Build history of the part. All positions in model axes, mm. A direction names the side the tool comes from. Round coordinates to 2 decimals unless told otherwise and drop trailing zeros. Write each loop counter-clockwise with the first axis right and the second up, starting at its lowest first coordinate (ties: lowest second). Pieces come first, ordered by that corner, then holes. Notation, with made-up numbers: (3, 85.25) - (12, 85.25) arc R24 cw to (12, 104.25) - close; hole circle Ø2 at (85.25, 82). An arc over 180 degrees is marked (long way). Answer as a JSON object with one key per item and string values. Group by question number.
Item 1: Slice it at C-C, the plane x = -51. List the corners of the cut face in (y, z).
Item 2: Two-plate mould, pull along X, no slides. Class faces 1 (the flat face through (-111.898, -38, -30)), 2 (the cylindrical face through (-23.18, -48.6, -16.73)), 3 (the cylindrical face through (-61.11, -37.23, -30.02)), 4 (the flat face through (-10.298, -39, -25)): +X half, -X half, draft (parallel to the pull), parting line (faces both ways), or undercut.
Item 3: Slice it at B-B, the plane y = -33.5. List the corners of the cut face in (x, z).
Item 4: Slice it at D-D, the plane y = -83. List the corners of the cut face in (x, z), then the cut area to 3 significant figures.
Item 5: Which spindle directions (+Z, -Z, +X, -X, +Y, -Y) get a long thin tool onto all of the face, cutting with end or side? Do faces 5 (the flat face through (-74, 0, -29)), 6 (the flat face through (-74, -83, -16.782)), 7 (the flat face through (-61.098, -83, -30)), 8 (the flat face through (-74, -83, -42.182)), 9 (the flat face through (-86.498, -83, -30)). Say none if no direction does.
Item 6: Flat gauge pins, fed straight in: pin 1 (11 mm diameter, centred on y = -85.5, z = -35, fed in from -X); pin 2 (15 mm diameter, centred on y = -82, z = -34, fed in from +X); pin 3 (4 mm diameter, centred on x = -80, y = -85, fed in from +Z). Where does each tip first touch, or does it go through?
Item 7: Probe line 1 (X direction, y = -37, z = -3); line 2 (X direction, y = -38, z = -14.5); line 3 (X direction, y = -71, z = -54). List the from-to ranges inside material, lowest first. Write a range as from..to.
Item 8: Slice it at A-A, the plane z = -19. List the corners of the cut face in (x, y), then the cut area to 3 significant figures.
from build123d import *

# Parameters (mm, degrees)
F0_W     = 76.2
F0_H     = 76.2
F1_DEPTH = 76.2
F3_D     = 25.4
F4_W     = 25.4
F4_H     = 25.4
F5_DEPTH = 13.462
F6_R     = 12.7
F7_DEPTH = 25.4
F8_DEPTH = 25.4


with BuildPart() as f1:
    # F0 (on Front) → F1 (new body)
    with BuildSketch(Plane.XZ):
        with Locations((-73.797528, -29.481855)):
            Rectangle(F0_W, F0_H)
    extrude(amount=F1_DEPTH)

    # F3 (through all)
    with Locations(Plane.XY.offset(8.618145)):
        with Locations((-73.797528, -37.791912)):
            Hole(F3_D / 2)

    # F4 (on face) → F5 (join)
    with BuildSketch(Plane.XZ.offset(76.2)):
        with Locations((-73.797528, -29.481855)):
            Rectangle(F4_W, F4_H)
    extrude(amount=F5_DEPTH)

    # F6 (on face) → F7 (join)
    with BuildSketch(Plane.YZ.offset(-35.697528)):
        with Locations((-39.237883, -25.310718)):
            Circle(F6_R)
    extrude(amount=F7_DEPTH)

    # F6 (on face) → F8 (join)
    with BuildSketch(Plane.YZ.offset(-35.697528)):
        with Locations((-39.237883, -25.310718)):
            Circle(F6_R)
    extrude(amount=F8_DEPTH)


solid = f1.part
Geometry says:
{
 "1": {"outline": "(-76.2, -67.58) - (0, -67.58) - (0, 8.62) - (-76.2, 8.62) - close"},
 "2": {"face 1": "-X half", "face 2": "draft", "face 3": "undercut", "face 4": "+X half"},
 "3": {"outline": "(-111.9, -67.58) - (-85.75, -67.58) - (-85.75, 8.62) - (-111.9, 8.62) - close; (-61.84, -67.58) - (-35.7, -67.58) - (-35.7, -36.64) - (-10.3, -36.64) - (-10.3, -13.98) - (-35.7, -13.98) - (-35.7, 8.62) - (-61.84, 8.62) - close"},
 "4": {"outline": "(-86.5, -42.18) - (-61.1, -42.18) - (-61.1, -16.78) - (-86.5, -16.78) - close", "area": "645 mm^2"},
 "5": {"face 5": "+Z, -Z, +X, -X, +Y", "face 6": "+Z, +X, -X, -Y", "face 7": "+Z, -Z, +X, -Y", "face 8": "-Z, +X, -X, -Y", "face 9": "+Z, -Z, -X, -Y"},
 "6": {"pin 1": "stops at x = -86.5", "pin 2": "stops at x = -35.7", "pin 3": "stops at z = -16.78"},
 "7": {"line 1": "x = -111.9..-86.47, -61.12..-35.7", "line 2": "x = -111.9..-86.5, -61.1..-10.3", "line 3": "x = -111.9..-35.7"},
 "8": {"outline": "(-111.9, -76.2) - (-86.5, -76.2) - (-86.5, -89.66) - (-61.1, -89.66) - (-61.1, -76.2) - (-35.7, -76.2) - (-35.7, -50.26) - (-10.3, -50.26) - (-10.3, -28.22) - (-35.7, -28.22) - (-35.7, 0) - (-111.9, 0) - close; hole circle Ø25.4 at (-73.8, -37.79)", "area": "6,200 mm^2"}
}
